Could you check a few things on this model? Use its own coordinates, in mm. Coordinates: 2 decimals unless noted, no trailing zeros. Loops run counter-clockwise (first coordinate to the right, second up) from the corner with the lowest first, then second, coordinate; pieces in that order, holes last. Notation, with made-up numbers: (-13.5, 59) - (17.5, 59) arc R14 ccw to (17.5, 69) - close; hole circle Ø5 at (78.5, 39.5). An arc over 180 degrees is marked (long way). One line per item, written item: value. Start each with the question number.
(1) I'm going to push flat-ended pins straight in: P1, Ø5, axis at x = 0, y = 2.5, coming from the -Z side; P2, Ø5, axis at x = -0.5, y = -1.5, coming from the +Z side; P3, Ø6, axis at y = -4, z = 5, coming from the +X side; P4, Ø3, axis at x = -4, z = 12, coming from the -Y side. Where does each tip first touch, or does it pass through?
(2) If we section it at C-C on z = 22.25: Write out the boundary of the cut face in (x, y), then the cut area to 3 significant figures.
(3) If I drill on line 1 along Y through (x, z) = (0, 21); line 2 along X through (y, z) = (1, 2.75), over which ranges is the centre line in solid material (lowest first)? Write a range as from..to.
(4) If we mould it in two halves opening along X, with no side actions, what happens to faces 1 (the face through (-6, 0, 15)), 2 (the face through (-1.42, -3.92, 0)), 3 (the face through (-0.867, -3.905, 14.544))? For each: pulls with the +X half, pulls with the -X half, needs draft (parallel to the pull), parting line crosses it, or undercut.
(5) If we section it at A-A on x = 0: Write out the boundary of the cut face in (y, z).
```python
from build123d import *

# Parameters (mm, degrees)
SKETCH_R        = 6
SKETCH_R_2      = 4
PAD_DEPTH       = 30
CHAMFER_SIZE    = 0.5
CHAMFER001_SIZE = 0.5


with BuildPart() as part:
    # Sketch → Pad (new body)
    with BuildSketch(Plane.XY):
        Circle(SKETCH_R)
        Circle(SKETCH_R_2, mode=Mode.SUBTRACT)
    extrude(amount=PAD_DEPTH)

    # Chamfer
    chamfer_edges = [part.edges().sort_by_distance(p)[0] for p in [
        (-4, 0, 30),
    ]]
    chamfer(chamfer_edges, length=CHAMFER_SIZE)

    # Chamfer001
    chamfer001_edges = [part.edges().sort_by_distance(p)[0] for p in [
        (-6, 0, 30),
    ]]
    chamfer(chamfer001_edges, length=CHAMFER001_SIZE)


solid = part.part
```
Values:
1. P1: stops at z = 0
1. P2: stops at z = 29.58
1. P3: stops at x = 5.92
1. P4: stops at y = -5.45
2. outline: circle Ø12 at (0, 0); hole circle Ø8 at (0, 0)
2. area: 62.8 mm2
3. line 1: y = -6..-4, 4..6
3. line 2: x = -5.92..-3.87, 3.87..5.92
4. face 1: parting line crosses it
4. face 2: needs draft
4. face 3: undercut
5. outline: (-6, 0) - (-4, 0) - (-4, 29.5) - (-4.5, 30) - (-5.5, 30) - (-6, 29.5) - close; (4, 0) - (6, 0) - (6, 29.5) - (5.5, 30) - (4.5, 30) - (4, 29.5) - close
